from build123d import *

# Parameters (mm, degrees)
F0_W     = 177.8
F0_H     = 177.8
F1_DEPTH = 101.6
F2_W     = 155.8
F2_H     = 79.6
F3_DEPTH = 177.801
F4_W     = 107.8
F4_H     = 31.6
F5_DEPTH = 177.801
F6_R     = 44.5
F7_DEPTH = 25


with BuildPart() as f1:
    # F0 (on Top) → F1 (new body)
    with BuildSketch(Plane.XY):
        with Locations((-7.112902, 1.270162)):
            Rectangle(F0_W, F0_H)
    extrude(amount=-F1_DEPTH)

    # F2 (on face) → F3 (cut, through all)
    with BuildSketch(Plane.XZ.offset(87.629838)):
        with Locations((-7.112902, -50.8)):
            Rectangle(F2_W, F2_H)
    extrude(amount=-F3_DEPTH, mode=Mode.SUBTRACT)

    # F4 (on face) → F5 (cut, through all)
    with BuildSketch(Plane(origin=(-96.012902, 0, 0), x_dir=(0, -1, 0), z_dir=(-1, 0, 0))):
        with Locations((-1.270162, -50.8)):
            Rectangle(F4_W, F4_H)
    extrude(amount=-F5_DEPTH, mode=Mode.SUBTRACT)

    # F6 (on face) → F7 (cut)
    with BuildSketch(Plane(origin=(0, 0, -101.6), x_dir=(1, 0, 0), z_dir=(0, 0, -1))):
        with Locations((-9.286336, 4.346757)):
            Circle(F6_R)
    extrude(amount=-F7_DEPTH, mode=Mode.SUBTRACT)


solid = f1.part
CAD build for the part. Positions are in the model's coordinates, mm. A direction names the side the tool comes from. Give positions to 0.01 mm unless a question says otherwise; leave off trailing zeros. Write each loop counter-clockwise with the first axis right and the second up, starting at its lowest first coordinate (ties: lowest second). Pieces come first, ordered by that corner, then holes. Notation, with made-up numbers: (85.5, 83) -> (111.5, 83) arc R31 ccw to (111.5, 119) -> close; hole circle Ø11 at (61.25, -13.5). An arc over 180 degrees is marked (long way). Return JSON: item names as keys, results as strings.
Item 1: Band-saw the part on A-A (z = -87). List the corners of the cut face in (x, y).
Answer below:
{"outline": "(-96.01, -87.63) -> (-85.01, -87.63) -> (-85.01, 90.17) -> (-96.01, 90.17) -> close; (70.79, -87.63) -> (81.79, -87.63) -> (81.79, 90.17) -> (70.79, 90.17) -> close"}
Item 2: Band-saw the part on C-C (z = -58.5). List the corners of the cut face in (x, y), then the cut area to 3 significant figures.
Answer below:
{"outline": "(-96.01, -87.63) -> (-85.01, -87.63) -> (-85.01, -52.63) -> (-96.01, -52.63) -> close; (-96.01, 55.17) -> (-85.01, 55.17) -> (-85.01, 90.17) -> (-96.01, 90.17) -> close; (70.79, -87.63) -> (81.79, -87.63) -> (81.79, -52.63) -> (70.79, -52.63) -> close; (70.79, 55.17) -> (81.79, 55.17) -> (81.79, 90.17) -> (70.79, 90.17) -> close", "area": "1,540 mm2"}
Item 3: Tool access for faces 4 (the flat face through (-8, 0, -11)), 5 (the flat face through (-91, 2, -35)), 6 (the cylindrical face through (-18.933, 39.095, -96.177)), 7 (the flat face through (-8, -87.63, -9)): list every direction of +Z, -Z, +X, -X, +Y, -Y with a clear straight run to the whole face (end or side of a thin tool).
Answer below:
{"face 4": "+Y, -Y", "face 5": "+X, -X", "face 6": "-Z", "face 7": "+Z, -Z, +X, -X, -Y"}
Item 4: Band-saw the part on B-B (x = 49). List the corners of the cut face in (y, z), then the cut area to 3 significant figures.
Answer below:
{"outline": "(-87.63, -101.6) -> (90.17, -101.6) -> (90.17, -90.6) -> (-87.63, -90.6) -> close; (-87.63, -11) -> (90.17, -11) -> (90.17, 0) -> (-87.63, 0) -> close", "area": "3,910 mm2"}
Item 5: Two-plate mould, pull along X, no slides. Class faces 1 (the flat face through (70.787, 0, -34)), 2 (the flat face through (-8, 3, 0)), 3 (the flat face through (81.787, 0, -28)): +X half, -X half, draft (parallel to the pull), parting line (faces both ways), or undercut.
Answer below:
{"face 1": "undercut", "face 2": "draft", "face 3": "+X half"}
Item 6: Drop a flat-ended pin along its axis: pin 1 (12 mm diameter, centred on x = 21.5, z = -11.5, fed in from +Y). Give the stop position or say it passes through.
Answer below:
{"pin 1": "stops at y = 90.17"}
Item 7: Drill centre lines: probe 1 along X at (y, z) = (-70, -51); probe 2 along Z at (x, y) = (57, 64.5); probe 3 along X at (y, z) = (-35, -94). Where is each one in solid material? Low to high.
Answer below:
{"probe 1": "x = -96.01 to -85.01, 70.79 to 81.79", "probe 2": "z = -101.6 to -90.6, -11 to 0", "probe 3": "x = -96.01 to -41.55, 22.97 to 81.79"}
Item 8: Band-saw the part on D-D (y = -67.5). List the corners of the cut face in (x, z), then the cut area to 3 significant figures.
Answer below:
{"outline": "(-96.01, -101.6) -> (81.79, -101.6) -> (81.79, 0) -> (-96.01, 0) -> close; hole (-85.01, -90.6) -> (70.79, -90.6) -> (70.79, -11) -> (-85.01, -11) -> close", "area": "5,660 mm2"}
